Answer from the drawing. Dimensions are ordinates in mm from the lowest x, y and z of the part. A direction names the side the tool comes from. Coordinates: 2 decimals unless noted, no trailing zeros. Write each loop counter-clockwise with the first axis right and the second up, starting at its lowest first coordinate (ties: lowest second). Pieces come first, ordered by that corner, then holes. Notation, with made-up numbers: (39, -16) -> (48, -16) arc R23 ccw to (48, 23) -> close; hole circle Ø11 at (-6, 86). An arc over 180 degrees is marked (long way). One line per item, written item: value. Start each with the question number.
1. Find section A-A, the plane y = 3.15. Write down the section's boundary in (x, z), and give its area (3 significant figures).
2. Given P1, Ø1.6, axis at x = 4.5, z = 8.5, coming from the +Y side; P2, Ø1, axis at y = 2, z = 3.5, coming from the +X side; P3, Ø0.8, axis at x = 2, z = 9, coming from the -Y side, each flat-ended and moving along its own axis, determine where each tip first touches the part or whether it passes through.
3. For a pull along Y with two mould halves and no side action, classify the marked faces 1, 2 and 3 as pulls with the +Y half, pulls with the -Y half, needs draft (parallel to the pull), parting line crosses it, or undercut.
4. For the marked faces 4 and 5, determine the directions among +Z, -Z, +X, -X, +Y, -Y from which every point of the face is accessible in a straight line to the end or side of a thin tool.
5. Consider line 1 along Z through (x, y) = (3.25, 1.5); line 2 along X through (y, z) = (3, 9); line 3 along X through (y, z) = (3.5, 8.5). Determine where each line is inside the solid, lowest interval first.
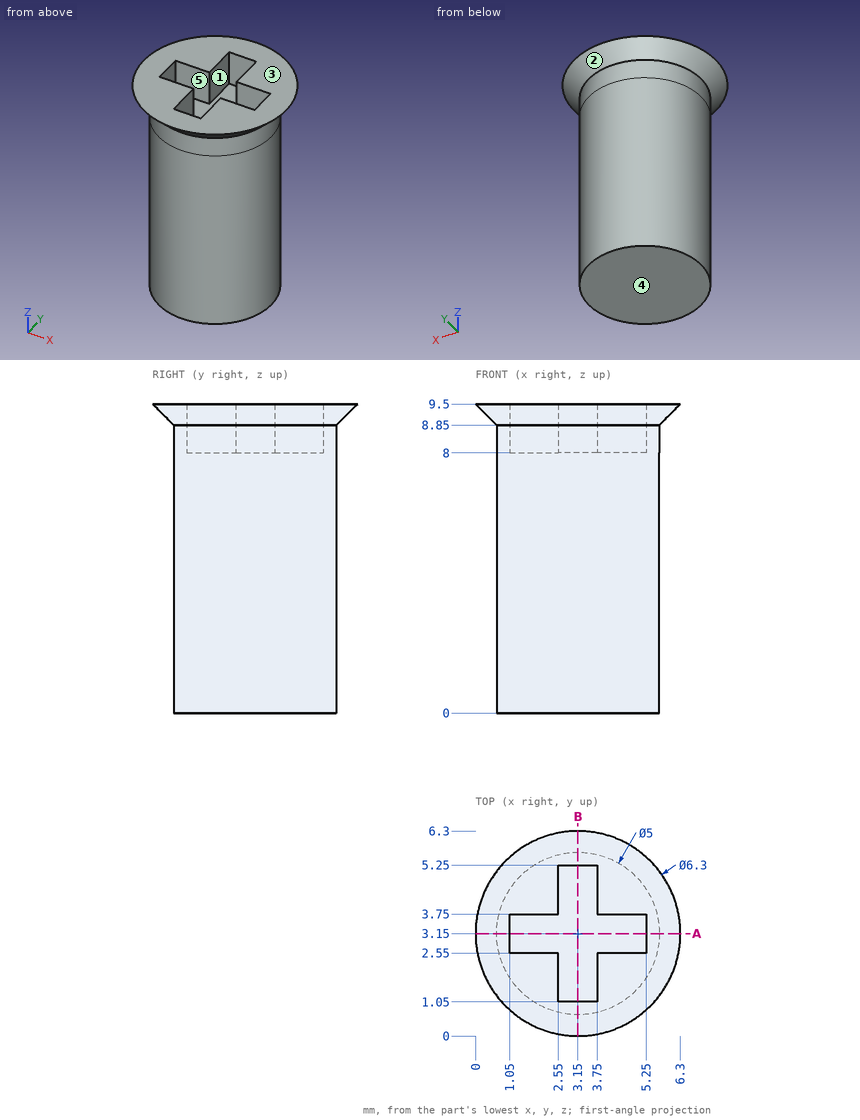
Answer block:
1. outline: (0, 9.5) -> (0.65, 8.85) -> (0.65, 0) -> (5.65, 0) -> (5.65, 8.85) -> (6.3, 9.5) -> (5.25, 9.5) -> (5.25, 8) -> (1.05, 8) -> (1.05, 9.5) -> close
1. area: 41.6 mm2
2. P1: stops at y = 5.84
2. P2: stops at x = 5.56
2. P3: stops at y = 0.3
3. face 1: undercut
3. face 2: parting line crosses it
3. face 3: needs draft
4. face 4: -Z, +X, -X, +Y, -Y
4. face 5: +Z
5. line 1: z = 0 to 8
5. line 2: x = 0.5 to 1.05, 5.25 to 5.8
5. line 3: x = 0.67 to 1.05, 5.25 to 5.63
